Here's how the part is built. I have some questions about the finished solid (model axes, mm). Face numbers are marked on the shaded views. Coordinates: 2 decimals unless noted, no trailing zeros. Write each loop counter-clockwise with the first axis right and the second up, starting at its lowest first coordinate (ties: lowest second). Pieces come first, ordered by that corner, then holes. Notation, with made-up numbers: M 76.5,36 L 105.5,36 A12 ccw 105.5,45 Z; hole C 1,-16 d4. An arc over 180 degrees is marked long. Use a Markdown table: item, result.
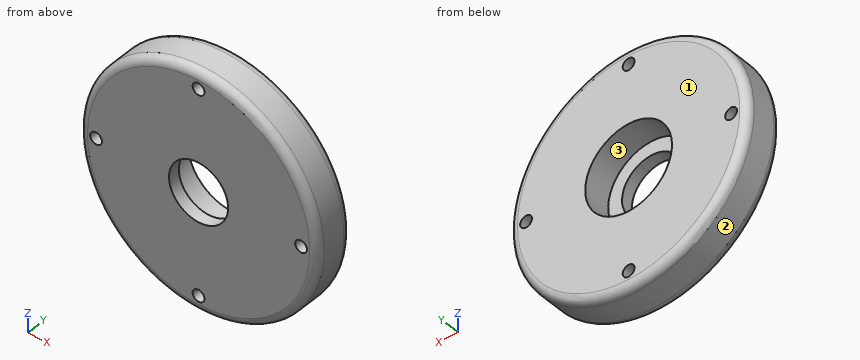
```python
from build123d import *

# Parameters (mm, degrees)
SKETCH1_R           = 30.18
SKETCH1_R_2         = 7.5
BOSS_EXTRUDE1_DEPTH = 10
SKETCH2_R           = 1.5
CUT_EXTRUDE1_DEPTH  = 44.836797328
SKETCH3_R           = 11
CUT_EXTRUDE2_DEPTH  = 7
FILLET1_R           = 2


with BuildPart() as part:
    # Sketch1 → Boss-Extrude1 (new body)
    with BuildSketch(Plane(origin=(0, 0, 0), x_dir=(1, 0, 0), z_dir=(0, 1, 0))):
        with Locations(Location((0, 0, 0), (0, 0, 270))):
            Circle(SKETCH1_R)
        with Locations(Location((0, 0, 0), (0, 0, 270))):
            Circle(SKETCH1_R_2, mode=Mode.SUBTRACT)
    extrude(amount=BOSS_EXTRUDE1_DEPTH)

    # Sketch2 → Cut-Extrude1 (cut, through all)
    with BuildSketch(Plane(origin=(0, 10, 0), x_dir=(1, 0, 0), z_dir=(0, 1, 0))):
        with Locations(Location((0, 26, 0), (0, 0, 270))):
            Circle(SKETCH2_R)
        with Locations(Location((26, 0, 0), (0, 0, 270))):
            Circle(SKETCH2_R)
        with Locations(Location((-26, 0, 0), (0, 0, 270))):
            Circle(SKETCH2_R)
        with Locations(Location((0, -26, 0), (0, 0, 270))):
            Circle(SKETCH2_R)
    extrude(amount=-CUT_EXTRUDE1_DEPTH, mode=Mode.SUBTRACT)

    # Sketch3 → Cut-Extrude2 (cut)
    with BuildSketch(Plane(origin=(0, 10, 0), x_dir=(1, 0, 0), z_dir=(0, 1, 0))):
        with Locations(Location((0, 0, 0), (0, 0, 270))):
            Circle(SKETCH3_R)
    extrude(amount=-CUT_EXTRUDE2_DEPTH, mode=Mode.SUBTRACT)

    # Fillet1
    fillet1_edges = [part.edges().sort_by_distance(p)[0] for p in [
        (0, 0, -30.18),
        (0, 10, -30.18),
    ]]
    fillet(fillet1_edges, radius=FILLET1_R)


solid = part.part
```
1. Suppose I cut it at A-A on x = 0. Write out the boundary of the cut face in (y, z).
Answers follow:
| item | result |
|---|---|
| outline | M 0,-28.18 A2 ccw 2,-30.18 L 8,-30.18 A2 ccw 10,-28.18 L 10,-27.5 L 0,-27.5 Z; M 0,-24.5 L 10,-24.5 L 10,-11 L 3,-11 L 3,-7.5 L 0,-7.5 Z; M 0,7.5 L 3,7.5 L 3,11 L 10,11 L 10,24.5 L 0,24.5 Z; M 0,27.5 L 10,27.5 L 10,28.18 A2 ccw 8,30.18 L 2,30.18 A2 ccw 0,28.18 Z |
2. We'd pull the mould along Z, two halves only. Please class the marked faces 1, 2 and 3: +Z half, -Z half, draft (parallel to the pull), parting line (faces both ways), or undercut.
Answers follow:
| item | result |
|---|---|
| face 1 | draft |
| face 2 | parting line |
| face 3 | undercut |
3. Suppose I cut it at C-C on y = 9.25. Write out the boundary of the cut face in (x, z), and give its area (3 significant figures).
Answers follow:
| item | result |
|---|---|
| outline | C 0,0 d59.48; hole C -26,0 d3; hole C 0,0 d22; hole C 0,-26 d3; hole C 0,26 d3; hole C 26,0 d3 |
| area | 2,370 mm2 |
4. Will these pins go through, and if not, where does the flat tip stop? pin 1 Ø6.5 at (x, z) = (4, 5) entering from +Y; pin 2 Ø3 at (x, y) = (14.5, 8) entering from -Z; pin 3 Ø2 at (y, z) = (4, 4) entering from +X.
Answers follow:
| item | result |
|---|---|
| pin 1 | stops at y = 3 |
| pin 2 | stops at z = -27.24 |
| pin 3 | stops at x = 30.03 |
5. Suppose I cut it at B-B on z = 0. Write out the boundary of the cut face in (x, y), and give its area (3 significant figures).
Answers follow:
| item | result |
|---|---|
| outline | M -30.18,2 A2 ccw -28.18,0 L -27.5,0 L -27.5,10 L -28.18,10 A2 ccw -30.18,8 Z; M -24.5,0 L -7.5,0 L -7.5,3 L -11,3 L -11,10 L -24.5,10 Z; M 7.5,0 L 24.5,0 L 24.5,10 L 11,10 L 11,3 L 7.5,3 Z; M 27.5,0 L 28.18,0 A2 ccw 30.18,2 L 30.18,8 A2 ccw 28.18,10 L 27.5,10 Z |
| area | 341 mm2 |
6. I need wall thicknesses on probe 1 along X at (y, z) = (3.25, 0); probe 2 along X at (y, z) = (1.95, 0); probe 3 along X at (y, z) = (8, 26). Which ranges of each line are inside material? Lowest first, please.
Answers follow:
| item | result |
|---|---|
| probe 1 | x = -30.18 to -27.5, -24.5 to -11, 11 to 24.5, 27.5 to 30.18 |
| probe 2 | x = -30.18 to -27.5, -24.5 to -7.5, 7.5 to 24.5, 27.5 to 30.18 |
| probe 3 | x = -15.32 to -1.5, 1.5 to 15.32 |
